from build123d import *

# Parameters (mm, degrees)
CROQUIS1_W              = 17.8
CROQUIS1_H              = 17.82
SALIENTE_EXTRUIR1_DEPTH = 143.52
CROQUIS2_W              = 11
CROQUIS2_H              = 143.52
CORTAR_EXTRUIR1_DEPTH   = 0.38
CROQUIS3_W              = 1.42
CROQUIS3_H              = 2
CORTAR_EXTRUIR2_DEPTH   = 144.52
CROQUIS4_W              = 4.77
CROQUIS4_H              = 5.05
CORTAR_EXTRUIR3_DEPTH   = 1
CORTAR_EXTRUIR4_START   = -142.52
CROQUIS5_W              = 4.77
CROQUIS5_H              = 5.05
CORTAR_EXTRUIR4_DEPTH   = 1
REDONDEO1_R             = 2.385
REDONDEO2_R             = 2.385
REDONDEO3_R             = 2.385
REDONDEO4_R             = 2.385
REDONDEO5_R             = 2.385
REDONDEO6_R             = 2.385
REDONDEO7_R             = 2.385
REDONDEO8_R             = 2.385
CROQUIS6_R              = 3.975
SALIENTE_EXTRUIR2_DEPTH = 1
CROQUIS7_R              = 2.95
CORTAR_EXTRUIR5_DEPTH   = 0.5
CROQUIS8_R              = 2.4
SALIENTE_EXTRUIR3_DEPTH = 117.49
SALIENTE_EXTRUIR4_DEPTH = 23.95
CROQUIS10_R             = 3.185
SALIENTE_EXTRUIR5_DEPTH = 4.95
CROQUIS15_R             = 4.92
SALIENTE_EXTRUIR6_DEPTH = 8


with BuildPart() as part:
    # Croquis1 → Saliente-Extruir1 (new body)
    with BuildSketch(Plane.XY):
        with Locations((8.9, 8.91)):
            Rectangle(CROQUIS1_W, CROQUIS1_H)
    extrude(amount=SALIENTE_EXTRUIR1_DEPTH)

    # Croquis2 → Cortar-Extruir1 (cut)
    with BuildSketch(Plane.XZ):
        with Locations((8.9, 71.76)):
            Rectangle(CROQUIS2_W, CROQUIS2_H)
    extrude(amount=-CORTAR_EXTRUIR1_DEPTH, mode=Mode.SUBTRACT)

    # Croquis3 → Cortar-Extruir2 (cut, through all)
    with BuildSketch(Plane(origin=(0, 0, 0), x_dir=(-1, 0, 0), z_dir=(0, 0, -1))):
        with Locations((-17.09, 3)):
            Rectangle(CROQUIS3_W, CROQUIS3_H)
        with Locations((-0.71, 3)):
            Rectangle(CROQUIS3_W, CROQUIS3_H)
    extrude(amount=-CORTAR_EXTRUIR2_DEPTH, mode=Mode.SUBTRACT)

    # Croquis4 → Cortar-Extruir3 (cut)
    with BuildSketch(Plane(origin=(0, 0, 0), x_dir=(-1, 0, 0), z_dir=(0, 0, -1))):
        with Locations((-2.385, 7.945)):
            Rectangle(CROQUIS4_W, CROQUIS4_H)
        with Locations((-15.415, 7.945)):
            Rectangle(CROQUIS4_W, CROQUIS4_H)
    extrude(amount=-CORTAR_EXTRUIR3_DEPTH, mode=Mode.SUBTRACT)

    # Croquis5 → Cortar-Extruir4 (cut)
    with BuildSketch(Plane(origin=(0, 0, 1), x_dir=(-1, 0, 0), z_dir=(0, 0, -1)).offset(CORTAR_EXTRUIR4_START)):
        with Locations((-15.415, 7.945)):
            Rectangle(CROQUIS5_W, CROQUIS5_H)
        with Locations((-2.385, 7.945)):
            Rectangle(CROQUIS5_W, CROQUIS5_H)
    extrude(amount=CORTAR_EXTRUIR4_DEPTH, mode=Mode.SUBTRACT)

    # Redondeo1
    redondeo1_edges = [part.edges().sort_by_distance(p)[0] for p in [
        (4.77, 5.42, 0.5),
    ]]
    fillet(redondeo1_edges, radius=REDONDEO1_R)

    # Redondeo2
    redondeo2_edges = [part.edges().sort_by_distance(p)[0] for p in [
        (4.77, 10.47, 0.5),
    ]]
    fillet(redondeo2_edges, radius=REDONDEO2_R)

    # Redondeo3
    redondeo3_edges = [part.edges().sort_by_distance(p)[0] for p in [
        (13.03, 10.47, 0.5),
    ]]
    fillet(redondeo3_edges, radius=REDONDEO3_R)

    # Redondeo4
    redondeo4_edges = [part.edges().sort_by_distance(p)[0] for p in [
        (13.03, 5.42, 0.5),
    ]]
    fillet(redondeo4_edges, radius=REDONDEO4_R)

    # Redondeo5
    redondeo5_edges = [part.edges().sort_by_distance(p)[0] for p in [
        (13.03, 10.47, 143.02),
    ]]
    fillet(redondeo5_edges, radius=REDONDEO5_R)

    # Redondeo6
    redondeo6_edges = [part.edges().sort_by_distance(p)[0] for p in [
        (13.03, 5.42, 143.02),
    ]]
    fillet(redondeo6_edges, radius=REDONDEO6_R)

    # Redondeo7
    redondeo7_edges = [part.edges().sort_by_distance(p)[0] for p in [
        (4.77, 5.42, 143.02),
    ]]
    fillet(redondeo7_edges, radius=REDONDEO7_R)

    # Redondeo8
    redondeo8_edges = [part.edges().sort_by_distance(p)[0] for p in [
        (4.77, 10.47, 143.02),
    ]]
    fillet(redondeo8_edges, radius=REDONDEO8_R)

    # Croquis6 → Saliente-Extruir2 (add)
    with BuildSketch(Plane.XY.offset(143.52)):
        with Locations((8.9, 9.1)):
            Circle(CROQUIS6_R)
    extrude(amount=SALIENTE_EXTRUIR2_DEPTH)

    # Croquis7 → Cortar-Extruir5 (cut)
    with BuildSketch(Plane.XY.offset(144.52)):
        with Locations((8.9, 9.1)):
            Circle(CROQUIS7_R)
    extrude(amount=-CORTAR_EXTRUIR5_DEPTH, mode=Mode.SUBTRACT)

    # Croquis8 → Saliente-Extruir3 (add)
    with BuildSketch(Plane.XY.offset(144.02)):
        with Locations((8.9, 9.1)):
            Circle(CROQUIS8_R)
    extrude(amount=SALIENTE_EXTRUIR3_DEPTH)

    # Croquis9 → Saliente-Extruir4 (add)
    with BuildSketch(Plane.XY.offset(261.51)):
        with BuildLine():
            Line((3.94, 4.145), (8.9, 4.145))
            Line((8.9, 4.145), (8.9, 6.7))
            ThreePointArc((8.9, 6.7), (6.5, 9.1), (8.9, 11.5))
            Line((8.9, 11.5), (8.9, 14.055))
            Line((8.9, 14.055), (3.94, 14.055))
            Line((3.94, 14.055), (3.94, 4.145))
        make_face()
        with BuildLine():
            Line((8.9, 6.7), (8.9, 4.145))
            Line((8.9, 4.145), (13.86, 4.145))
            Line((13.86, 4.145), (13.86, 14.055))
            Line((13.86, 14.055), (8.9, 14.055))
            Line((8.9, 14.055), (8.9, 11.5))
            ThreePointArc((8.9, 11.5), (10.597056275, 10.797056275), (11.3, 9.1))
            ThreePointArc((11.3, 9.1), (10.597056275, 7.402943725), (8.9, 6.7))
        make_face()
        with BuildLine():
            ThreePointArc((8.9, 11.5), (6.5, 9.1), (8.9, 6.7))
            Line((8.9, 6.7), (8.9, 11.5))
        make_face()
        with BuildLine():
            Line((8.9, 11.5), (8.9, 6.7))
            ThreePointArc((8.9, 6.7), (10.597056275, 7.402943725), (11.3, 9.1))
            ThreePointArc((11.3, 9.1), (10.597056275, 10.797056275), (8.9, 11.5))
        make_face()
    extrude(amount=SALIENTE_EXTRUIR4_DEPTH)

    # Croquis10 → Saliente-Extruir5 (add)
    with BuildSketch(Plane(origin=(0, 0, 0), x_dir=(-1, 0, 0), z_dir=(0, 0, -1))):
        with Locations((-8.9, 8.91)):
            Circle(CROQUIS10_R)
    extrude(amount=SALIENTE_EXTRUIR5_DEPTH)

    # Croquis15 → Saliente-Extruir6 (add)
    with BuildSketch(Plane(origin=(0, 0, -4.95), x_dir=(-1, 0, 0), z_dir=(0, 0, -1))):
        with Locations((-8.9, 8.91)):
            Circle(CROQUIS15_R)
    extrude(amount=SALIENTE_EXTRUIR6_DEPTH)


solid = part.part
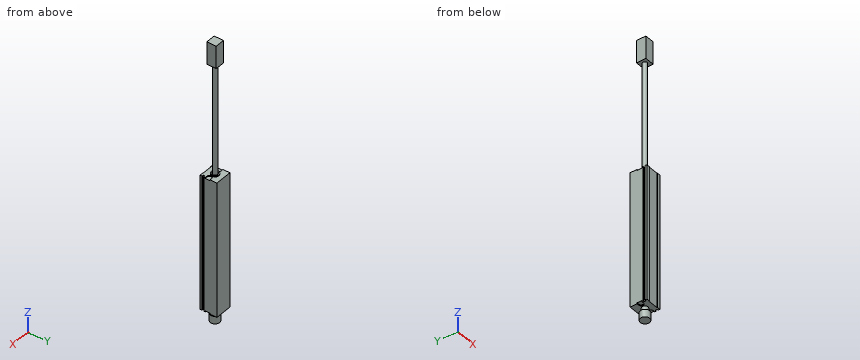
The listing builds one solid part. Answer for the finished solid, in the listing's coordinates (mm). Coordinates: 2 decimals unless noted, no trailing zeros. Loops run counter-clockwise (first coordinate to the right, second up) from the corner with the lowest first, then second, coordinate; pieces in that order, holes last. Notation, with made-up numbers: (33.5, 25) -> (44.5, 25) arc R26 cw to (44.5, 56) -> close; hole circle Ø1 at (33, 37.25). An arc over 180 degrees is marked (long way). Answer in a Markdown table with one row per item. Add a question column.
1. Flat-ended cylindrical pins translate along their axes: P1, Ø2.5, axis at x = 16.5, y = 7.5, coming from the -Z side; P2, Ø8, axis at y = 10, z = 278.5, coming from the +X side; P3, Ø1, axis at x = 16, y = 15, coming from the +Z side. Find the tip coordinate at first contact, or state that the pin passes through.
2. The part is cut by section A-A, the plane x = 8.9. Write down the section's boundary in (y, z) (3 decimals), then the cut area to 3 significant figures.
3. The part is cut by section B-B, the plane z = 15. Write down the section's boundary in (x, y).
4. The part is cut by section C-C, the plane z = 179. Write down the section's boundary in (x, y).
5. Consider line 1 (Y direction, x = 8.9, z = 144.4) (3 decimals); line 2 (Y direction, x = 5, z = 264) (3 decimals); line 3 (Z direction, x = 14.25, y = 12.75). Determine where each line is inside the solid, lowest interval first. Write a range as [from, to].
Answer below:
| question | item | result |
|---|---|---|
| 1 | P1 | z = 1 |
| 1 | P2 | x = 13.86 |
| 1 | P3 | z = 143.52 |
| 2 | outline | (0.38, 0) -> (5.725, 0) -> (5.725, -4.95) -> (3.99, -4.95) -> (3.99, -12.95) -> (13.83, -12.95) -> (13.83, -4.95) -> (12.095, -4.95) -> (12.095, 0) -> (17.82, 0) -> (17.82, 143.52) -> (13.075, 143.52) -> (13.075, 144.52) -> (12.05, 144.52) -> (12.05, 144.02) -> (11.5, 144.02) -> (11.5, 261.51) -> (14.055, 261.51) -> (14.055, 285.46) -> (4.145, 285.46) -> (4.145, 261.51) -> (6.7, 261.51) -> (6.7, 144.02) -> (6.15, 144.02) -> (6.15, 144.52) -> (5.125, 144.52) -> (5.125, 143.52) -> (0.38, 143.52) -> close |
| 2 | area | 3,420 mm2 |
| 3 | outline | (0, 0) -> (3.4, 0) -> (3.4, 0.38) -> (14.4, 0.38) -> (14.4, 0) -> (17.8, 0) -> (17.8, 2) -> (16.38, 2) -> (16.38, 4) -> (17.8, 4) -> (17.8, 17.82) -> (0, 17.82) -> (0, 4) -> (1.42, 4) -> (1.42, 2) -> (0, 2) -> close |
| 4 | outline | circle Ø4.8 at (8.9, 9.1) |
| 5 | line 1 | [5.125, 6.15], [6.7, 11.5], [12.05, 13.075] |
| 5 | line 2 | [4.145, 14.055] |
| 5 | line 3 | [0, 143.52] |
